Verification items for the finished model (mm, model axes). Coordinates: 2 decimals unless noted, no trailing zeros. Order: outer loops, then holes, each group sorted by start corner. A loop starts at its lowest first (then second) coordinate and runs counter-clockwise, first axis right, second up. Notation, with made-up numbers: (-38, -7) -> (-2, -7) arc R10 cw to (-2, 4) -> close; hole circle Ø6 at (30, 14.25). An arc over 180 degrees is marked (long way). Write item = value, one per line. Start each with the question number.
1. Cross-section at B-B on y = 43. Record the cut outline in (x, z), plus the area to 3 significant figures.
2. Thickness scan on line 1 along X through (y, z) = (3, -3.55); line 2 along X through (y, z) = (27.5, -2.4); line 3 along Y through (x, z) = (55.5, -2.6). Record the ranges inside material, lowest first. Write a range as from..to.
3. Cross-section at A-A on x = 78. Record the cut outline in (y, z), plus the area to 3 significant figures.
4. Go/stop test with flat-tipped pins: P1, Ø1.2, axis at x = 48.5, z = -3, coming from the +Y side; P2, Ø2, axis at x = 84.5, z = -2, coming from the -Y side; P3, Ø10, axis at x = 13, y = 25, coming from the +Z side; P4, Ø1.2, axis at y = 23.5, z = -2.5, coming from the +X side. Record where each tip stops, or that it passes through.
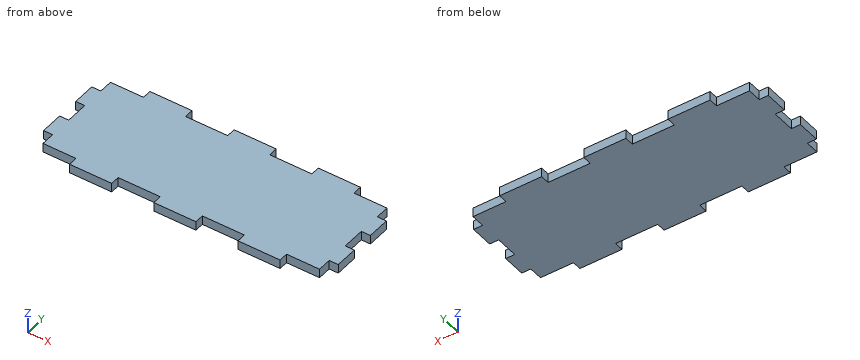
from build123d import *

# Parameters (mm, degrees)
BUITENAFMETING_RECHTHOEK_W  = 130
BUITENAFMETING_RECHTHOEK_H  = 50
PLAAT_DEPTH                 = 4
TAND_HOR_W                  = 18.571428571
TAND_HOR_H                  = 4
TAND_BOVEN_DEPTH            = 5
TANDEN_PATROON_BOVEN_COUNT  = 4
TANDEN_PATROON_BOVEN_PITCH  = 37.142857143
TAND_VER_W                  = 4
TAND_VER_H                  = 10
TAND_LINKS_DEPTH            = 5
TANDEN_PATROON_LINKS_COUNT  = 3
TANDEN_PATROON_LINKS_PITCH  = 20
TAND_O_W                    = 18.571428571
TAND_O_H                    = 4
TAND_ONDER_DEPTH            = 5
TANDEN_PATROON_ONDER_COUNT  = 4
TANDEN_PATROON_ONDER_PITCH  = 37.142857143
TAND_R_W                    = 4
TAND_R_H                    = 10
TAND_RECHTS_DEPTH           = 5
TANDEN_PATROON_RECHTS_COUNT = 3
TANDEN_PATROON_RECHTS_PITCH = 20


with BuildPart() as part:
    # Buitenafmeting Rechthoek → Plaat (new body)
    with BuildSketch(Plane.XY):
        with Locations((65, 25)):
            Rectangle(BUITENAFMETING_RECHTHOEK_W, BUITENAFMETING_RECHTHOEK_H)
    extrude(amount=-PLAAT_DEPTH)

    # Tand Hor → Tand Boven (cut, through all)
    with BuildSketch(Plane.XY):
        with Locations((9.285714286, 48)):
            Rectangle(TAND_HOR_W, TAND_HOR_H)
    tand_boven = extrude(amount=-TAND_BOVEN_DEPTH, mode=Mode.SUBTRACT)

    # Tanden Patroon Boven: Tand Boven ×4
    with Locations(*[(i * TANDEN_PATROON_BOVEN_PITCH, 0, 0) for i in range(1, TANDEN_PATROON_BOVEN_COUNT)]):
        add(tand_boven, mode=Mode.SUBTRACT)

    # Tand Ver → Tand Links (cut, through all)
    with BuildSketch(Plane.XY):
        with Locations((2, 45)):
            Rectangle(TAND_VER_W, TAND_VER_H)
    tand_links = extrude(amount=-TAND_LINKS_DEPTH, mode=Mode.SUBTRACT)

    # Tanden Patroon Links: Tand Links ×3
    with Locations(*[(0, -i * TANDEN_PATROON_LINKS_PITCH, 0) for i in range(1, TANDEN_PATROON_LINKS_COUNT)]):
        add(tand_links, mode=Mode.SUBTRACT)

    # Tand O → Tand Onder (cut, through all)
    with BuildSketch(Plane.XY):
        with Locations((9.285714286, 2)):
            Rectangle(TAND_O_W, TAND_O_H)
    tand_onder = extrude(amount=-TAND_ONDER_DEPTH, mode=Mode.SUBTRACT)

    # Tanden Patroon Onder: Tand Onder ×4
    with Locations(*[(i * TANDEN_PATROON_ONDER_PITCH, 0, 0) for i in range(1, TANDEN_PATROON_ONDER_COUNT)]):
        add(tand_onder, mode=Mode.SUBTRACT)

    # Tand R → Tand Rechts (cut, through all)
    with BuildSketch(Plane.XY):
        with Locations((128, 45)):
            Rectangle(TAND_R_W, TAND_R_H)
    tand_rechts = extrude(amount=-TAND_RECHTS_DEPTH, mode=Mode.SUBTRACT)

    # Tanden Patroon Rechts: Tand Rechts ×3
    with Locations(*[(0, -i * TANDEN_PATROON_RECHTS_PITCH, 0) for i in range(1, TANDEN_PATROON_RECHTS_COUNT)]):
        add(tand_rechts, mode=Mode.SUBTRACT)


solid = part.part
Worked out:
q1.outline = (4, -4) -> (126, -4) -> (126, 0) -> (4, 0) -> close
q1.area = 488 mm²
q2.line_1 = 18.57..37.14, 55.71..74.29, 92.86..111.43
q2.line_2 = 4..126
q2.line_3 = 4..46
q3.outline = (4, -4) -> (46, -4) -> (46, 0) -> (4, 0) -> close
q3.area = 168 mm²
q4.P1 = 46
q4.P2 = 4
q4.P3 = 0
q4.P4 = 126
